The listing builds one solid part. Answer for the finished solid, in the listing's coordinates (mm). A direction names the side the tool comes from. Coordinates: 2 decimals unless noted, no trailing zeros. Order: outer loops, then holes, each group sorted by start corner. A loop starts at its lowest first (then second) coordinate and runs counter-clockwise, first axis right, second up. Notation, with made-up numbers: (83, 79) -> (103, 79) arc R24 ccw to (103, 108) -> close; hole circle Ø1 at (87, -14). An arc over 180 degrees is marked (long way). Answer in a Markdown table with one row per item. Add a question column.
```python
from build123d import *

# Parameters (mm, degrees)
SKETCH1_W           = 100
SKETCH1_H           = 40
BOSS_EXTRUDE1_DEPTH = 15
MOVE_FACE4_BY       = 5
SKETCH5_R           = 10
CUT_EXTRUDE2_DEPTH  = 2
MOVE_FACE5_BY       = 7.5
MOVE_FACE5_2_BY     = 7.5
MOVE_FACE7_BY       = 75
MOVE_FACE8_BY       = 5
MOVE_FACE9_BY       = 12.7
SKETCH6_W           = 15
SKETCH6_H           = 10
BOSS_EXTRUDE2_DEPTH = 100
MOVE_FACE10_BY      = 22.5
SKETCH7_W           = 15
SKETCH7_H           = 77.5
BOSS_EXTRUDE3_DEPTH = 47.8
MOVE_FACE11_BY      = 5
MOVE_FACE12_BY      = 6.7
MOVE_FACE13_BY      = 4.1
MOVE_FACE16_BY      = 0.9
MOVE_FACE17_BY      = 10
MOVE_FACE18_BY      = 10


with BuildPart() as part:
    # Sketch1 → Boss-Extrude1 (new body)
    with BuildSketch(Plane(origin=(0, 0, 0), x_dir=(1, 0, 0), z_dir=(0, 1, 0))):
        Rectangle(SKETCH1_W, SKETCH1_H)
    extrude(amount=BOSS_EXTRUDE1_DEPTH)

    # Move Face4: a face moved outward by 5.0
    extrude(part.faces().sort_by_distance((50, 7.5, 0))[0], amount=MOVE_FACE4_BY, dir=(1, 0, 0))

    # Sketch5 → Cut-Extrude2 (cut)
    with BuildSketch(Plane(origin=(0, 15, 0), x_dir=(1, 0, 0), z_dir=(0, 1, 0))):
        with Locations(Location((40, 0, 0), (0, 0, 270))):
            Circle(SKETCH5_R)
    extrude(amount=-CUT_EXTRUDE2_DEPTH, mode=Mode.SUBTRACT)

    # Move Face5: a face moved inward by 7.5
    extrude(part.faces().sort_by_distance((2.5, 7.5, -20))[0], amount=MOVE_FACE5_BY, dir=(0, 0, 1), mode=Mode.SUBTRACT)

    # Move Face5 2: a face moved inward by 7.5
    extrude(part.faces().sort_by_distance((2.5, 7.5, 20))[0], amount=MOVE_FACE5_2_BY, dir=(0, 0, -1), mode=Mode.SUBTRACT)

    # Move Face7: a face moved inward by 75.0
    extrude(part.faces().sort_by_distance((-50, 7.5, 0))[0], amount=MOVE_FACE7_BY, dir=(1, 0, 0), mode=Mode.SUBTRACT)

    # Move Face8: a face moved inward by 5.0
    extrude(part.faces().sort_by_distance((40, 0, 0))[0], amount=MOVE_FACE8_BY, dir=(0, 1, 0), mode=Mode.SUBTRACT)

    # Move Face9: a face moved outward by 12.7
    extrude(part.faces().sort_by_distance((55, 10, 0))[0], amount=MOVE_FACE9_BY, dir=(1, 0, 0))

    # Sketch6 → Boss-Extrude2 (add)
    with BuildSketch(Plane(origin=(0, 0, -12.5), x_dir=(-1, 0, 0), z_dir=(0, 0, -1))):
        with Locations((-60.2, 10)):
            Rectangle(SKETCH6_W, SKETCH6_H)
    extrude(amount=BOSS_EXTRUDE2_DEPTH)

    # Move Face10: a face moved inward by 22.5
    extrude(part.faces().sort_by_distance((60.2, 10, -112.5))[0], amount=MOVE_FACE10_BY, dir=(0, 0, 1), mode=Mode.SUBTRACT)

    # Sketch7 → Boss-Extrude3 (add)
    with BuildSketch(Plane(origin=(0, 15, 0), x_dir=(1, 0, 0), z_dir=(0, 1, 0))):
        with Locations((60.2, 51.25)):
            Rectangle(SKETCH7_W, SKETCH7_H)
    extrude(amount=BOSS_EXTRUDE3_DEPTH)

    # Move Face11: a face moved inward by 5.0
    extrude(part.faces().sort_by_distance((53.570011211, 5, -26.716647982))[0], amount=MOVE_FACE11_BY, dir=(0, 1, 0), mode=Mode.SUBTRACT)

    # Move Face12: a face moved inward by 6.7
    extrude(part.faces().sort_by_distance((60.2, 62.8, -51.25))[0], amount=MOVE_FACE12_BY, dir=(0, -1, 0), mode=Mode.SUBTRACT)

    # Move Face13: a face moved outward by 4.1
    extrude(part.faces().sort_by_distance((60.2, 56.1, -51.25))[0], amount=MOVE_FACE13_BY, dir=(0, 1, 0))

    # Move Face16: a face moved outward by 0.9
    extrude(part.faces().sort_by_distance((60.2, 60.2, -51.25))[0], amount=MOVE_FACE16_BY, dir=(0, 1, 0))

    # Move Face17: a face moved inward by 10.0
    extrude(part.faces().sort_by_distance((60.2, 38.05, -12.5))[0], amount=MOVE_FACE17_BY, dir=(0, 0, -1), mode=Mode.SUBTRACT)

    # Move Face18: a face moved inward by 10.0
    extrude(part.faces().sort_by_distance((60.2, 35.55, -90))[0], amount=MOVE_FACE18_BY, dir=(0, 0, 1), mode=Mode.SUBTRACT)


solid = part.part
```
Q1. A cutting plane is placed at D-D (x = 51.5). Determine the outline of the cut face in (y, z), then the cut area to 3 significant figures.
Q2. A cutting plane is placed at A-A (x = 40). Determine the outline of the cut face in (y, z), then the cut area to 3 significant figures.
Q3. A cutting plane is placed at C-C (y = 26). Determine the outline of the cut face in (x, z).
Q4. Straight lines are drawn through the part: line 1 (X direction, y = 13.7, z = 0); line 2 (Y direction, x = 64.5, z = -20); line 3 (Z direction, x = 55, y = 35.5). For each, find the intervals that lie inside material, in ascending order.
Q5. Given pin 1 (4 mm diameter, centred on y = 44.5, z = -61, fed in from -X); pin 2 (10.5 mm diameter, centred on x = 39.5, z = -10, fed in from +Y); pin 3 (12 mm diameter, centred on x = 59, y = 45, fed in from +Z), each flat-ended and moving along its own axis, determine where each tip first touches the part or whether it passes through.
Q6. For faces 5 (the face through (52.7, 35, -46)), 6 (the face through (46, 12, 12.5)), 7 (the face through (30.24, 14.01, -2.17)), 8 (the face through (51, 15, -1)), determine the directions among +Z, -Z, +X, -X, +Y, -Y from which every point of the face is accessible in a straight line to the end or side of a thin tool.
Q7. A cutting plane is placed at B-B (z = 0). Determine the outline of the cut face in (x, y).
Q8. Determine the mould class of faces 1 (the face through (39, 12, -12.5)), 2 (the face through (40, 13, 0)), 3 (the face through (67.7, 35, -43)), 4 (the face through (60, 38, -22.5)) for opening direction Z: +Z half, -Z half, draft (parallel to the pull), parting line (faces both ways), or undercut.
Returned:
| question | item | result |
|---|---|---|
| 1 | outline | (10, -12.5) -> (15, -12.5) -> (15, 12.5) -> (10, 12.5) -> close |
| 1 | area | 125 mm² |
| 2 | outline | (10, -12.5) -> (15, -12.5) -> (15, -10) -> (13, -10) -> (13, 10) -> (15, 10) -> (15, 12.5) -> (10, 12.5) -> close |
| 2 | area | 85.0 mm² |
| 3 | outline | (52.7, -80) -> (67.7, -80) -> (67.7, -22.5) -> (52.7, -22.5) -> close |
| 4 | line 1 | x = 25 to 30, 50 to 67.7 |
| 4 | line 2 | y = 10 to 15 |
| 4 | line 3 | z = -80 to -22.5 |
| 5 | pin 1 | stops at x = 52.7 |
| 5 | pin 2 | stops at y = 15 |
| 5 | pin 3 | stops at z = -22.5 |
| 6 | face 5 | -Z, -X, +Y, -Y |
| 6 | face 6 | +Z, +X, -X, +Y, -Y |
| 6 | face 7 | +Y |
| 6 | face 8 | +Z, +X, -X, +Y |
| 7 | outline | (25, 10) -> (67.7, 10) -> (67.7, 15) -> (50, 15) -> (50, 13) -> (30, 13) -> (30, 15) -> (25, 15) -> close |
| 8 | face 1 | -Z half |
| 8 | face 2 | undercut |
| 8 | face 3 | draft |
| 8 | face 4 | +Z half |
